Input: part model. Units: mm. Frame: model coordinates. A direction names the side the tool comes from. Coordinates: 2 decimals unless noted, no trailing zeros. Loops run counter-clockwise (first coordinate to the right, second up) from the corner with the lowest first, then second, coordinate; pieces in that order, holes last. Notation, with made-up numbers: (-10, 36) -> (3, 36) arc R25 cw to (3, 62) -> close; hole circle Ø4 at (88, 10.25). An arc over 180 degrees is marked (long way). Put each result on its own line as item: value. Start each with the question number.
1) Contact query for flat-ended pins moving along their axis: P1, Ø3, axis at x = -38.5, y = -2, coming from the +Z side; P2, Ø6.5, axis at x = -193.5, z = 361.5, coming from the +Y side; P3, Ø9, axis at y = 65.5, z = -201, coming from the +X side. Output: stop coordinate, or through.
2) Set-up query: faces 4 (the flat face through (178.06, -38.24, 822.62)), 5 (the flat face through (-193.94, 37.62, 823.24)), 6 (the flat face through (178.06, 38.24, -822.62)). Return all of +Z, -Z, +X, -X, +Y, -Y with unobstructed straight access to the full face (end or side cutting, diameter ignored); none if empty.
3) Cut plane C-C (z = -12.5). Return the cut outline in (x, y).
4) Cut plane D-D (z = -352.5). Return the cut outline in (x, y), plus the area to 3 significant figures.
5) Pull-direction query (Y, two-part tool) for faces 1 (the cylindrical face through (168.82, -3.36, 820.13)), 2 (the flat face through (-193.94, -38.24, 822.62)), 3 (the flat face through (178.06, 37.62, 823.24)); classes: pulls with the +Y half, pulls with the -Y half, needs draft (parallel to the pull), parting line crosses it, or undercut.
6) Cut plane A-A (z = -705). State how many separate pieces and enclosed holes the cut face has, plus the area to 3 significant figures.
7) Material intervals for L1, parallel to Y at x = 153.5, z = 462.5; L2, parallel to X at y = 17.5, z = 289; L3, parallel to Y at x = 172, z = 805, sorted ascending.
8) Cut plane B-B (x = 70). Return the cut outline in (y, z), plus the area to 3 significant figures.
from build123d import *

# Parameters (mm, degrees)
EXTRUDE_1_DEPTH        = 855
EXTRUDE_2_DEPTH        = 10
SKETCH_3_W             = 350
SKETCH_3_H             = 6
EXTRUDE_3_DEPTH        = 174
CUT_EXTRUDE_9_DEPTH    = 932.891088057
EXTRUDE_7_DEPTH        = 8
PATTERN_LINEAR_1_COUNT = 2
PATTERN_LINEAR_1_PITCH = 372
SKETCH_9_R             = 15.5
CUT_EXTRUDE_10_DEPTH   = 939.256361556


with BuildPart() as part:
    # 草图1 → 拉伸1 (new body)
    with BuildSketch(Plane.XY):
        Polygon((-150, 70), (-190, 70), (-190, -70), (-150, -70), (-150, -62), (-182, -62), (-182, 62), (-150, 62), align=None)
    extrude(amount=EXTRUDE_1_DEPTH)

    # 草图2 → 拉伸2 (add)
    with BuildSketch(Plane(origin=(-182, 0, 0), x_dir=(0, 0, -1), z_dir=(1, 0, 0))):
        with BuildLine():
            Line((-676.539819016, 62), (-855, 62))
            Line((-855, 62), (-855, -62))
            Line((-855, -62), (-676.539819016, -62))
            ThreePointArc((-676.539819016, -62), (-655, 0), (-676.539819016, 62))
        make_face()
    extrude(amount=EXTRUDE_2_DEPTH)

    # 草图3 → 拉伸3 (add)
    with BuildSketch(Plane(origin=(-182, 0, 0), x_dir=(0, 0, -1), z_dir=(1, 0, 0))):
        with Locations((-460, -1)):
            Rectangle(SKETCH_3_W, SKETCH_3_H)
    extrude(amount=EXTRUDE_3_DEPTH)

    # 镜向1: part across plane


with BuildPart() as part_1:
    add(part.part)
    add(part.part.mirror(Plane(origin=(-8, -4, 635), x_dir=(0, 0, 1), z_dir=(1, 0, 0))))

    # 草图8 → 拉伸9 (cut, through all)
    with BuildSketch(Plane.ZY.offset(190)):
        Polygon((805, 70), (855, 70), (855, 20), align=None)
        Polygon((855, -70), (855, -20), (805, -70), align=None)
    extrude(amount=-CUT_EXTRUDE_9_DEPTH, mode=Mode.SUBTRACT)

    # 镜向2: part across plane


with BuildPart() as part_2:
    add(part_1.part)
    add(part_1.part.mirror(Plane.XY))

    # 草图6 → 拉伸7 (add)
    with BuildSketch(Plane.ZY.offset(190)):
        Polygon((-800.857864376, 60), (-845, 15.857864376), (-845, -15.857864376), (-800.857864376, -60), (800.857864376, -60), (845, -15.857864376), (845, 15.857864376), (800.857864376, 60), align=None)
    extrude_7 = extrude(amount=EXTRUDE_7_DEPTH)

    # 阵列(线性)1: 拉伸7 ×2
    with Locations(*[(i * PATTERN_LINEAR_1_PITCH, 0, 0) for i in range(1, PATTERN_LINEAR_1_COUNT)]):
        add(extrude_7)

    # 草图9 → 拉伸10 (cut, through all)
    with BuildSketch(Plane.ZY.offset(198)):
        with Locations((-805, 0)):
            Circle(SKETCH_9_R)
        with Locations((-705, 0)):
            Circle(SKETCH_9_R)
        with Locations(Location((705, 0, 0), (0, 0, 90))):
            Circle(SKETCH_9_R)
        with Locations(Location((805, 0, 0), (0, 0, 90))):
            Circle(SKETCH_9_R)
    extrude(amount=-CUT_EXTRUDE_10_DEPTH, mode=Mode.SUBTRACT)


solid = part_2.part
Results found:
1. P1: stops at z = 635
1. P2: stops at y = 60
1. P3: stops at x = 174
2. face 4: +Z, +X, -Y
2. face 5: +Z, -X, +Y
2. face 6: -Z, +X, +Y
3. outline: (-198, -60) -> (-190, -60) -> (-190, -70) -> (-150, -70) -> (-150, -62) -> (-182, -62) -> (-182, 62) -> (-150, 62) -> (-150, 70) -> (-190, 70) -> (-190, 60) -> (-198, 60) -> close; (134, -70) -> (174, -70) -> (174, -60) -> (182, -60) -> (182, 60) -> (174, 60) -> (174, 70) -> (134, 70) -> (134, 62) -> (166, 62) -> (166, -62) -> (134, -62) -> close
4. outline: (-198, -60) -> (-190, -60) -> (-190, -70) -> (-150, -70) -> (-150, -62) -> (-182, -62) -> (-182, -4) -> (166, -4) -> (166, -62) -> (134, -62) -> (134, -70) -> (174, -70) -> (174, -60) -> (182, -60) -> (182, 60) -> (174, 60) -> (174, 70) -> (134, 70) -> (134, 62) -> (166, 62) -> (166, 2) -> (-182, 2) -> (-182, 62) -> (-150, 62) -> (-150, 70) -> (-190, 70) -> (-190, 60) -> (-198, 60) -> close
4. area: 7,270 mm2
5. face 1: undercut
5. face 2: pulls with the -Y half
5. face 3: pulls with the +Y half
6. separate pieces: 4
6. enclosed holes: 0
6. area: 6,050 mm2
7. L1: y = -70 to -62, -4 to 2, 62 to 70
7. L2: x = -198 to -182, 166 to 182
7. L3: y = -70 to -15.5, 15.5 to 70
8. outline: (-4, -635) -> (2, -635) -> (2, -285) -> (-4, -285) -> close; (-4, 285) -> (2, 285) -> (2, 635) -> (-4, 635) -> close
8. area: 4,200 mm2
